```python
from build123d import *

# Parameters (mm, degrees)
CROQUIS1_W              = 100.6
CROQUIS1_H              = 55
SALIENTE_EXTRUIR1_DEPTH = 2
CROQUIS2_W              = 100.6
CROQUIS2_H              = 2
SALIENTE_EXTRUIR2_DEPTH = 70
SALIENTE_EXTRUIR3_DEPTH = 100.6
CROQUIS4_W              = 10
CROQUIS4_H              = 5.6
CROQUIS4_W_2            = 20
CROQUIS4_H_2            = 20
CORTAR_EXTRUIR1_DEPTH   = 1.414213562
CROQUIS5_R              = 1.5
CORTAR_EXTRUIR2_DEPTH   = 2
CROQUIS6_W              = 60
CROQUIS6_H              = 2
SALIENTE_EXTRUIR4_DEPTH = 60
SALIENTE_EXTRUIR5_REACH = 181.856
CROQUIS7_W              = 2
CROQUIS7_H              = 10.5
CROQUIS8_W              = 64
CROQUIS8_H              = 2
SALIENTE_EXTRUIR6_DEPTH = 10.5
CROQUIS9_W              = 10
CROQUIS9_H              = 2
SALIENTE_EXTRUIR7_DEPTH = 2
CROQUIS10_W             = 10
CROQUIS10_H             = 5.6
CORTAR_EXTRUIR3_DEPTH   = 11
CORTAR_EXTRUIR4_DEPTH   = 10


with BuildPart() as part:
    # Croquis1 → Saliente-Extruir1 (new body)
    with BuildSketch(Plane(origin=(0, 0, 0), x_dir=(1, 0, 0), z_dir=(0, 1, 0))):
        Rectangle(CROQUIS1_W, CROQUIS1_H)
    extrude(amount=SALIENTE_EXTRUIR1_DEPTH)

    # Croquis2 → Saliente-Extruir2 (add)
    with BuildSketch(Plane(origin=(0, 0, 0), x_dir=(-1, 0, 0), z_dir=(0, -1, 0))):
        with Locations((0, -28.5)):
            Rectangle(CROQUIS2_W, CROQUIS2_H)
    extrude(amount=-SALIENTE_EXTRUIR2_DEPTH)

    # Croquis3 → Saliente-Extruir3 (add)
    with BuildSketch(Plane(origin=(50.3, 0, 0), x_dir=(0, 0, -1), z_dir=(1, 0, 0))):
        Polygon((-29.5, 70), (27.5, 127), (27.5, 125), (-27.5, 70), align=None)
    extrude(amount=-SALIENTE_EXTRUIR3_DEPTH)

    # Croquis4 → Cortar-Extruir1 (cut)
    with BuildSketch(Plane(origin=(0, 49.75, 49.75), x_dir=(1, 0, 0), z_dir=(0, 0.7071067811865513, 0.7071067811865438))):
        with Locations((0, 31.437824638)):
            Rectangle(CROQUIS4_W, CROQUIS4_H)
        with Locations((0, 68.942911166)):
            Rectangle(CROQUIS4_W_2, CROQUIS4_H_2)
    extrude(amount=-CORTAR_EXTRUIR1_DEPTH, mode=Mode.SUBTRACT)

    # Croquis5 → Cortar-Extruir2 (cut)
    with BuildSketch(Plane.XY.offset(29.5)):
        with Locations((0, 51)):
            Circle(CROQUIS5_R)
    extrude(amount=-CORTAR_EXTRUIR2_DEPTH, mode=Mode.SUBTRACT)

    # Croquis6 → Saliente-Extruir4 (add)
    with BuildSketch(Plane.XY.offset(29.5)):
        with Locations((0, 60.5)):
            Rectangle(CROQUIS6_W, CROQUIS6_H)
    extrude(amount=SALIENTE_EXTRUIR4_DEPTH)

    # Saliente-Extruir5: up to this face of the body (flat: up to its plane)
    saliente_extruir5_end = Plane(part.part.faces().sort_by_distance((0, 34.541123817, 29.5))[0])
    # Croquis7 → Saliente-Extruir5 (add, up to the picked face)
    with BuildSketch(Plane.XY.offset(89.5), mode=Mode.PRIVATE) as saliente_extruir5_sk1:
        with Locations((31, 64.75)):
            Rectangle(CROQUIS7_W, CROQUIS7_H)
    saliente_extruir5_tool1 = split(extrude(saliente_extruir5_sk1.sketch, amount=-SALIENTE_EXTRUIR5_REACH, mode=Mode.PRIVATE), bisect_by=saliente_extruir5_end, keep=Keep.BOTH, mode=Mode.PRIVATE)
    # Croquis7 → Saliente-Extruir5 (add, up to the picked face)
    with BuildSketch(Plane.XY.offset(89.5), mode=Mode.PRIVATE) as saliente_extruir5_sk2:
        with Locations((-31, 64.75)):
            Rectangle(CROQUIS7_W, CROQUIS7_H)
    saliente_extruir5_tool2 = split(extrude(saliente_extruir5_sk2.sketch, amount=-SALIENTE_EXTRUIR5_REACH, mode=Mode.PRIVATE), bisect_by=saliente_extruir5_end, keep=Keep.BOTH, mode=Mode.PRIVATE)
    add(saliente_extruir5_tool1.solids().sort_by(Axis((31, 64.75, 89.5), (0, 0, -1)))[0])
    add(saliente_extruir5_tool2.solids().sort_by(Axis((-31, 64.75, 89.5), (0, 0, -1)))[0])

    # Croquis8 → Saliente-Extruir6 (add)
    with BuildSketch(Plane(origin=(0, 59.5, 0), x_dir=(-1, 0, 0), z_dir=(0, -1, 0))):
        with Locations((0, -90.5)):
            Rectangle(CROQUIS8_W, CROQUIS8_H)
    extrude(amount=-SALIENTE_EXTRUIR6_DEPTH)

    # Croquis9 → Saliente-Extruir7 (add)
    with BuildSketch(Plane(origin=(0, 0, 27.5), x_dir=(-1, 0, 0), z_dir=(0, 0, -1))):
        with Locations((0, 69)):
            Rectangle(CROQUIS9_W, CROQUIS9_H)
    extrude(amount=-SALIENTE_EXTRUIR7_DEPTH)

    # Croquis10 → Cortar-Extruir3 (cut)
    with BuildSketch(Plane.XY.offset(29.5)):
        with Locations((0, 72.8)):
            Rectangle(CROQUIS10_W, CROQUIS10_H)
    extrude(amount=-CORTAR_EXTRUIR3_DEPTH, mode=Mode.SUBTRACT)

    # Croquis11 → Cortar-Extruir4 (cut)
    with BuildSketch(Plane.XY.offset(29.5)):
        Polygon((0, 75.6), (7.15, 75.6), (7.15, 70), (-7.15, 70), (-7.15, 75.6), align=None)
    extrude(amount=-CORTAR_EXTRUIR4_DEPTH, mode=Mode.SUBTRACT)


solid = part.part
```
Geometry check sheet. Reference: the model listing, model coordinates, mm. A direction names the side the tool comes from. Give positions to 0.01 mm unless a question says otherwise; leave off trailing zeros. Order: outer loops, then holes, each group sorted by start corner. A loop starts at its lowest first (then second) coordinate and runs counter-clockwise, first axis right, second up. Notation, with made-up numbers: (-6.75, 18.5) - (21.25, 18.5) arc R22 ccw to (21.25, 31.5) - close; hole circle Ø1 at (-4.75, 50). An arc over 180 degrees is marked (long way). Answer in a Markdown table with one row per item. Add a question column.
Q1. Tool access check on faces 1 (the flat face through (0, 70, 90)), 2 (the flat face through (-30, 66, 60)), 3 (the flat face through (1, 36, 27.5)). Record the directions out of +Z, -Z, +X, -X, +Y, -Y that give a thin tool (end or side, any length) a straight path to the whole face; none if there is none.
Q2. Cross-section at B-B, the plane z = 38. Enter the section's corners in (x, y), then the cut area to 3 significant figures.
Q3. Gauge pin test, flat ends, axial feed: pin 1 (2.5 mm diameter, centred on x = 3.5, y = 67, fed in from -Z); pin 2 (12 mm diameter, centred on x = -19.5, z = 17, fed in from +Y); pin 3 (4 mm diameter, centred on x = -27.5, y = 32.5, fed in from +Z); pin 4 (0.6 mm diameter, centred on x = 2, z = 22.5, fed in from -Y). Record the tip position at first contact, or that the pin passes through.
Q4. Mould release check, pull along Y, two halves, no side actions. Record for faces 4 (the flat face through (1, 0, 1)), 5 (the flat face through (11.9, 97.9, -0.4)), 6 (the flat face through (0, 66, 29.5)), 7 (the flat face through (0, 61.5, 59)): pulls with the +Y half, pulls with the -Y half, needs draft (parallel to the pull), parting line crosses it, or undercut.
Q5. Cross-section at A-A, the plane x = -18. Enter the section's corners in (y, z).
Q6. Cross-section at D-D, the plane x = 43.5. Enter the section's corners in (y, z).
Q7. Material ranges on probe 1 along Y at (x, z) = (0, 28); probe 2 along Y at (x, z) = (12, 46); probe 3 along Z at (x, y) = (-22.5, 33), recorded low to high. Write a range as from..to.
Q8. Cross-section at C-C, the plane y = 109. Enter the section's corners in (x, z), then the cut area to 3 significant figures.
Check values:
| question | item | result |
|---|---|---|
| 1 | face 1 | +Z, +X, -X, +Y |
| 1 | face 2 | +Y |
| 1 | face 3 | -Z, +X, -X |
| 2 | outline | (-32, 59.5) - (32, 59.5) - (32, 70) - (30, 70) - (30, 61.5) - (-30, 61.5) - (-30, 70) - (-32, 70) - close |
| 2 | area | 162 mm^2 |
| 3 | pin 1 | stops at z = 27.5 |
| 3 | pin 2 | stops at y = 88.5 |
| 3 | pin 3 | stops at z = 29.5 |
| 3 | pin 4 | stops at y = 0 |
| 4 | face 4 | pulls with the -Y half |
| 4 | face 5 | undercut |
| 4 | face 6 | needs draft |
| 4 | face 7 | pulls with the +Y half |
| 5 | outline | (0, -27.5) - (2, -27.5) - (2, 27.5) - (70, 27.5) - (125, -27.5) - (127, -27.5) - (70, 29.5) - (61.5, 29.5) - (61.5, 89.5) - (70, 89.5) - (70, 91.5) - (59.5, 91.5) - (59.5, 29.5) - (0, 29.5) - close |
| 6 | outline | (0, -27.5) - (2, -27.5) - (2, 27.5) - (70, 27.5) - (125, -27.5) - (127, -27.5) - (70, 29.5) - (0, 29.5) - close |
| 7 | probe 1 | y = 0..49.5, 52.5..70 |
| 7 | probe 2 | y = 59.5..61.5 |
| 7 | probe 3 | z = 27.5..29.5 |
| 8 | outline | (-50.3, -11.5) - (50.3, -11.5) - (50.3, -9.5) - (-50.3, -9.5) - close |
| 8 | area | 201 mm^2 |
